from build123d import *

# Parameters (mm, degrees)
BOSS_EXTRUDE1_DEPTH     = 10
FILLET1_R               = 2
SKETCH2_R               = 1
CUT_EXTRUDE1_DEPTH      = 6
CUT_EXTRUDE1_DEPTH_BACK = 3
FILLET2_R               = 1


with BuildPart() as part:
    # Sketch1 → Boss-Extrude1 (new body)
    with BuildSketch(Plane(origin=(0, 0, 0), x_dir=(0, 0, -1), z_dir=(1, 0, 0))):
        Polygon((-2.75, 0), (-7.75, 0), (-7.75, -4), (-13.75, -4), (-13.75, -2), (-9.75, -2), (-9.75, 3), (9.75, 3), (9.75, -2), (13.75, -2), (13.75, -4), (7.75, -4), (7.75, 0), (2.75, 0), (2.75, -1.3), (-2.75, -1.3), align=None)
    extrude(amount=BOSS_EXTRUDE1_DEPTH)

    # Fillet1
    fillet1_edges = [part.edges().sort_by_distance(p)[0] for p in [
        (0, -3, 13.75),
        (0, -3, -13.75),
        (5, 3, 9.75),
        (5, 3, -9.75),
        (10, -3, -13.75),
        (10, -3, 13.75),
    ]]
    fillet(fillet1_edges, radius=FILLET1_R)

    # Sketch2 → Cut-Extrude1 (cut, two sides)
    with BuildSketch(Plane(origin=(0, -2, 0), x_dir=(1, 0, 0), z_dir=(0, 1, 0))) as cut_extrude1_sk:
        with Locations((8, -11.75)):
            Circle(SKETCH2_R)
        with Locations((2, -11.75)):
            Circle(SKETCH2_R)
        with Locations((2, 11.75)):
            Circle(SKETCH2_R)
        with Locations((8, 11.75)):
            Circle(SKETCH2_R)
    extrude(amount=CUT_EXTRUDE1_DEPTH, mode=Mode.SUBTRACT)
    extrude(cut_extrude1_sk.sketch, amount=-CUT_EXTRUDE1_DEPTH_BACK, mode=Mode.SUBTRACT)

    # Fillet2
    fillet2_edges = [part.edges().sort_by_distance(p)[0] for p in [
        (5, 0, 2.75),
        (5, 0, 7.75),
        (5, 0, -7.75),
        (5, 0, -2.75),
    ]]
    fillet(fillet2_edges, radius=FILLET2_R)


solid = part.part
Source: CAD feature listing. Evaluate the final solid. Frame: model axes, mm. A direction names the side the tool comes from. Coordinates: 2 decimals unless noted, no trailing zeros. Loops run counter-clockwise (first coordinate to the right, second up) from the corner with the lowest first, then second, coordinate; pieces in that order, holes last. Notation, with made-up numbers: (85.5, 76.25) - (140.5, 76.25) arc R6 cw to (140.5, 87.25) - close; hole circle Ø9 at (43, 44.25). An arc over 180 degrees is marked (long way). One line per item, written item: value. Start each with the question number.
1. Ray query, L1, parallel to X at y = -3.4, z = 11.75; L2, parallel to Z at x = 8, y = -2.6; L3, parallel to Z at x = 8, y = -1.5. Return the intervals inside material, ascending.
2. Section C-C (z = 11). Return the cut outline in (x, y), and give its area (3 significant figures).
3. Set-up query: faces 5 (the flat face through (5, -2, 12)), 6 (the cylindrical face through (5.07, -0.301, -3.035)), 7 (the flat face through (5, -2, -12)), 8 (the cylindrical face through (7.263, -2.986, 11.074)). Return all of +Z, -Z, +X, -X, +Y, -Y with unobstructed straight access to the full face (end or side cutting, diameter ignored); none if empty.
4. Section D-D (z = -2.25). Return the cut outline in (x, y).
5. Section B-B (x = 5). Return the cut outline in (y, z), and give its area (3 significant figures).
6. Section A-A (y = -2.5). Return the cut outline in (x, z), and give its area (3 significant figures).
7. Contact query for flat-ended pins moving along their axis: P1, Ø4, axis at x = 4, y = 2, coming from the -Z side; P2, Ø3, axis at x = 5, z = 1, coming from the -Y side; P3, Ø2, axis at x = 2.5, y = 1, coming from the +Z side. Output: stop coordinate, or through.
8. Mould query, pull axis X, two halves, no side actions, for faces 1 (the cylindrical face through (1.263, -2.986, 11.074)), 2 (the flat face through (5, -3, 13.75)), 3 (the cylindrical face through (9.4, -2.99, 13.18)), 4 (the flat face through (0, 0, 0)). Classes: pulls with the +X half, pulls with the -X half, needs draft (parallel to the pull), parting line crosses it, or undercut.
Verdict:
1. L1: x = 0 to 1, 3 to 7, 9 to 10
1. L2: z = -13.75 to -12.75, -10.75 to -7.75, 7.75 to 10.75, 12.75 to 13.75
1. L3: z = -9.75 to -7.75, 7.75 to 9.75
2. outline: (0, -4) - (1.34, -4) - (1.34, -2) - (0, -2) - close; (2.66, -4) - (7.34, -4) - (7.34, -2) - (2.66, -2) - close; (8.66, -4) - (10, -4) - (10, -2) - (8.66, -2) - close
2. area: 14.7 mm2
3. face 5: +Z, +X, -X, +Y
3. face 6: +X, -X, -Y
3. face 7: -Z, +X, -X, +Y
3. face 8: +Y, -Y
4. outline: (0, -1.3) - (10, -1.3) - (10, 3) - (0, 3) - close
5. outline: (-4, -13.75) - (-2, -13.75) - (-2, -9.75) - (1, -9.75) arc R2 ccw to (3, -7.75) - (3, 7.75) arc R2 ccw to (1, 9.75) - (-2, 9.75) - (-2, 13.75) - (-4, 13.75) - (-4, 7.75) - (-1, 7.75) arc R1 cw to (0, 6.75) - (0, 3.75) arc R1 cw to (-1, 2.75) - (-1.3, 2.75) - (-1.3, -2.75) - (-1, -2.75) arc R1 cw to (0, -3.75) - (0, -6.75) arc R1 cw to (-1, -7.75) - (-4, -7.75) - close
5. area: 96.8 mm2
6. outline: (0, -11.75) arc R2 ccw to (2, -13.75) - (8, -13.75) arc R2 ccw to (10, -11.75) - (10, -7.75) - (0, -7.75) - close; (0, 7.75) - (10, 7.75) - (10, 11.75) arc R2 ccw to (8, 13.75) - (2, 13.75) arc R2 ccw to (0, 11.75) - close; hole circle Ø2 at (2, -11.75); hole circle Ø2 at (2, 11.75); hole circle Ø2 at (8, -11.75); hole circle Ø2 at (8, 11.75)
6. area: 104 mm2
7. P1: stops at z = -9.75
7. P2: stops at y = -1.3
7. P3: stops at z = 9.75
8. face 1: undercut
8. face 2: needs draft
8. face 3: pulls with the +X half
8. face 4: pulls with the -X half
